```python
from build123d import *

# Parameters (mm, degrees)
SKETCH1_R                            = 20
BOSS_EXTRUDE1_DEPTH                  = 10
SKETCH1_R_2                          = 40
SKETCH1_R_3                          = 36
BOSS_EXTRUDE1_2_DEPTH                = 10
BOSS_EXTRUDE2_REACH                  = 89.446
BOSS_EXTRUDE2_END_RADIUS             = 36
BOSS_EXTRUDE2_START                  = 30
BOSS_EXTRUDE2_DIRECTION_2_REACH      = 89.446
BOSS_EXTRUDE2_DIRECTION_2_END_RADIUS = 20
CIRPATTERN1_COUNT                    = 12
SKETCH5_R                            = 1.735695499
BOSS_EXTRUDE3_DEPTH                  = 5
SCALE1_SCALE                         = 0.75
SKETCH6_R                            = 30
SKETCH6_R_2                          = 27
BOSS_EXTRUDE4_DEPTH                  = 100


with BuildPart() as part:
    # Sketch1 → Boss-Extrude1 (new body)
    with BuildSketch(Plane(origin=(0, 0, 0), x_dir=(1, 0, 0), z_dir=(0, 1, 0))):
        with Locations(Location((0, 0, 0), (0, 0, 270))):
            Circle(SKETCH1_R)
    extrude(amount=BOSS_EXTRUDE1_DEPTH)


with BuildPart() as body_2:
    # Sketch1 → Boss-Extrude1 2 (new body)
    with BuildSketch(Plane(origin=(0, 0, 0), x_dir=(1, 0, 0), z_dir=(0, 1, 0))):
        with Locations(Location((0, 0, 0), (0, 0, 270))):
            Circle(SKETCH1_R_2)
        with Locations(Location((0, 0, 0), (0, 0, 270))):
            Circle(SKETCH1_R_3, mode=Mode.SUBTRACT)
    extrude(amount=BOSS_EXTRUDE1_2_DEPTH)


    add(part.part)  # Boss-Extrude2 merges part
    # Boss-Extrude2: up to this cylinder (the profile starts inside it)
    boss_extrude2_end = Plane(origin=(0, 5, 0), z_dir=(0, -1, 0)) * Cylinder(BOSS_EXTRUDE2_END_RADIUS, 251.892, mode=Mode.PRIVATE)
    # Sketch4 → Boss-Extrude2 (add, up to the surface)
    with BuildSketch(Plane(origin=(0, 0, 0), x_dir=(0, 0, -1), z_dir=(1, 0, 0)).offset(BOSS_EXTRUDE2_START), mode=Mode.PRIVATE) as boss_extrude2_sk1:
        Polygon((-4.262410526, 0), (4.031443844, 10), (5.315133993, 10), (-2.978720377, 0), align=None)
    boss_extrude2_tool1 = extrude(boss_extrude2_sk1.sketch, amount=BOSS_EXTRUDE2_REACH, mode=Mode.PRIVATE) & boss_extrude2_end
    boss_extrude2 = boss_extrude2_tool1.solids().sort_by_distance((30, 5, -0.526362))[0]
    add(boss_extrude2)

    # Boss-Extrude2 direction 2: up to this cylinder (the profile starts outside it)
    boss_extrude2_direction_2_end = Plane(origin=(0, 5, 0), z_dir=(0, -1, 0)) * Cylinder(BOSS_EXTRUDE2_DIRECTION_2_END_RADIUS, 219.892, mode=Mode.PRIVATE)
    # Sketch4 → Boss-Extrude2 direction 2 (add, up to the surface)
    with BuildSketch(Plane(origin=(0, 0, 0), x_dir=(0, 0, -1), z_dir=(1, 0, 0)).offset(BOSS_EXTRUDE2_START), mode=Mode.PRIVATE) as boss_extrude2_direction_2_sk1:
        Polygon((-4.262410526, 0), (4.031443844, 10), (5.315133993, 10), (-2.978720377, 0), align=None)
    boss_extrude2_direction_2_tool1 = extrude(boss_extrude2_direction_2_sk1.sketch, amount=-BOSS_EXTRUDE2_DIRECTION_2_REACH, mode=Mode.PRIVATE) - boss_extrude2_direction_2_end
    boss_extrude2_direction_2 = boss_extrude2_direction_2_tool1.solids().sort_by_distance((30, 5, -0.526362))[0]
    add(boss_extrude2_direction_2)
    boss_extrude2 = boss_extrude2 + boss_extrude2_direction_2  # both directions under the feature's name, for the pattern or mirror that repeats it

    # CirPattern1: Boss-Extrude2 ×12 about axis
    cirpattern1_axis = Axis((0, 0, 0), (0, 1, 0))
    for i in range(1, CIRPATTERN1_COUNT):
        add(boss_extrude2.rotate(cirpattern1_axis, i * 360 / CIRPATTERN1_COUNT))

    # Sketch5 → Boss-Extrude3 (add)
    with BuildSketch(Plane(origin=(0, 10, 0), x_dir=(1, 0, 0), z_dir=(0, 1, 0))):
        with Locations(Location((-14.887021655, 0, 0), (0, 0, 270))):
            Circle(SKETCH5_R)
        with Locations(Location((-7.443510827, 12.89253894, 0), (0, 0, 270))):
            Circle(SKETCH5_R)
        with Locations(Location((7.443510827, 12.89253894, 0), (0, 0, 270))):
            Circle(SKETCH5_R)
        with Locations(Location((14.887021655, 0, 0), (0, 0, 270))):
            Circle(SKETCH5_R)
        with Locations(Location((7.443510827, -12.89253894, 0), (0, 0, 270))):
            Circle(SKETCH5_R)
        with Locations(Location((-7.443510827, -12.89253894, 0), (0, 0, 270))):
            Circle(SKETCH5_R)
    extrude(amount=BOSS_EXTRUDE3_DEPTH)


with BuildPart() as body_2_1:
    # Scale1: scaled about (0, 0, 0)
    add(body_2.part.scale(SCALE1_SCALE))

    # Sketch6 → Boss-Extrude4 (add)
    with BuildSketch(Plane(origin=(0, 7.5, 0), x_dir=(1, 0, 0), z_dir=(0, 1, 0))):
        with Locations(Location((0, 0, 0), (0, 0, 270))):
            Circle(SKETCH6_R)
        with Locations(Location((0, 0, 0), (0, 0, 85.253793096))):
            Circle(SKETCH6_R_2, mode=Mode.SUBTRACT)
    extrude(amount=BOSS_EXTRUDE4_DEPTH)


solid = body_2_1.part
```
Check sheet for the modelled part. Datum: model origin and axes. Units: mm. A direction names the side the tool comes from. Coordinates: 2 decimals unless noted, no trailing zeros. Order: outer loops, then holes, each group sorted by start corner. A loop starts at its lowest first (then second) coordinate and runs counter-clockwise, first axis right, second up. Notation, with made-up numbers: (50, -4.5) -> (54, -4.5) arc R34 cw to (54, 31.5) -> close; hole circle Ø8 at (35.5, -5.5). An arc over 180 degrees is marked (long way). Write item = value, one per line. Start each with the question number.
1) Go/stop test with flat-tipped pins: P1, Ø6, axis at y = 59, z = -3.5, coming from the +X side; P2, Ø1.3, axis at x = 11, z = -0.5, coming from the +Y side; P3, Ø4, axis at x = -15.5, y = 48, coming from the -Z side. Record where each tip stops, or that it passes through.
2) Access from +Z, -Z, +X, -X, +Y, -Y to the whole of each face (thin tool, end or side, straight path). Record for faces 1 (the flat face through (18.337, 3.803, 9.525)), 2 (the cylindrical face through (4.2, 3.7, 14.4)), 3 (the flat face through (-20.74, 3.7, -0.13)).
3) Cross-section at C-C (z = 0). Enter the section's corners in (x, y).
4) Cross-section at A-A (x = 0). Enter the section's corners in (y, z), then the cut area to 3 significant figures.
5) Cross-section at B-B (y = 57). Enter the section's corners in (x, z).
6) Material ranges on L1, parallel to X at y = 65, z = 0; L2, parallel to Z at x = 15.5, y = 71.5; L3, parallel to X at y = 103.5, z = -13, recorded low to high.
Ans:
q1.P1 = 30
q1.P2 = 11.25
q1.P3 = -26.79
q2.face_1 = -Y
q2.face_2 = none
q2.face_3 = +Y
q3.outline = (-30, 0) -> (-27, 0) -> (-27, 2.69) -> (-15, 2.69) -> (-15, 0) -> (15, 0) -> (15, 2.69) -> (27, 2.69) -> (27, 0) -> (30, 0) -> (30, 107.5) -> (27, 107.5) -> (27, 3.85) -> (15, 3.85) -> (15, 7.5) -> (12.47, 7.5) -> (12.47, 11.25) -> (9.86, 11.25) -> (9.86, 7.5) -> (-9.86, 7.5) -> (-9.86, 11.25) -> (-12.47, 11.25) -> (-12.47, 7.5) -> (-15, 7.5) -> (-15, 3.85) -> (-27, 3.85) -> (-27, 107.5) -> (-30, 107.5) -> close
q4.outline = (0, -30) -> (107.5, -30) -> (107.5, -27) -> (3.85, -27) -> (3.85, -15) -> (7.5, -15) -> (7.5, 15) -> (3.85, 15) -> (3.85, 27) -> (107.5, 27) -> (107.5, 30) -> (0, 30) -> (0, 27) -> (2.69, 27) -> (2.69, 15) -> (0, 15) -> (0, -15) -> (2.69, -15) -> (2.69, -27) -> (0, -27) -> close
q4.area = 898 mm²
q5.outline = circle Ø60 at (0, 0); hole circle Ø54 at (0, 0)
q6.L1 = -30 to -27, 27 to 30
q6.L2 = -25.69 to -22.11, 22.11 to 25.69
q6.L3 = -27.04 to -23.66, 23.66 to 27.04
